Read the model definition and answer for the solid it produces. Units are mm, in the model's axes. A direction names the side the tool comes from. Coordinates: 2 decimals unless noted, no trailing zeros. Loops run counter-clockwise (first coordinate to the right, second up) from the corner with the lowest first, then second, coordinate; pieces in that order, holes last.
Q1. The mould has two halves that part along Y. Classify faces 4 (the face through (105.966, 292.984, 121.478)), 5 (the face through (205.07, -8.67, -39.05)), 6 (the face through (210, -5, 73)): pulls with the +Y half, pulls with the -Y half, needs draft (parallel to the pull), parting line crosses it, or undercut.
Q2. Section A-A (z = 0) is taken. Give the vertices of the cut face in (x, y).
Q3. Straight lines are drawn through the part: line 1 (Z direction, x = 147, y = 0); line 2 (X direction, y = 305.5, z = 112); line 3 (Y direction, x = 119, z = -268). For each, find the intervals that lie inside material, in ascending order.
Q4. Section C-C (x = 78) is taken. Give the vertices of the cut face in (y, z).
Q5. Flat-ended cylindrical pins translate along their axes: P1, Ø12, axis at x = 118, z = -73.5, coming from the +Y side; P2, Ø1.5, axis at y = -227.5, z = -124.5, coming from the -X side; P3, Ø2, axis at x = 63.5, y = 254.5, coming from the +Z side; P4, Ø5, axis at y = -206.5, z = 242.5, coming from the -X side. Find the tip coordinate at first contact, or state that the pin passes through.
Q6. Which of the six approach directions +Z, -Z, +X, -X, +Y, -Y give full straight-line access (tool end or side, diameter ignored) to faces 1 (the face through (174.75, -68.92, 310.36)), 2 (the face through (200, 4, -62)), 3 (the face through (0, -258, -157))?
from build123d import *

# Parameters (mm, degrees)
SKETCH2_R          = 300
CUT_EXTRUDE1_DEPTH = 200
SKETCH3_R          = 40
CUT_EXTRUDE2_DEPTH = 200


with BuildPart() as part:
    # Sketch1 → Revolve2 (revolve)
    with BuildSketch(Plane.XY):
        Polygon((0, 0), (0, 350), (12, 329.169330118), (24, 329.169330118), (36, 317.169330118), (174, 317.169330118), (186, 329.169330118), (198, 329.169330118), (210, 350), (210, 0), align=None)
    revolve(axis=Axis((210, 0, 0), (-1, 0, 0)))

    # Sketch2 → Cut-Extrude1 (cut)
    with BuildSketch(Plane.ZY):
        with Locations(Location((0, 0, 0), (0, 0, 270))):
            Circle(SKETCH2_R)
    extrude(amount=-CUT_EXTRUDE1_DEPTH, mode=Mode.SUBTRACT)

    # Sketch3 → Cut-Extrude2 (cut)
    with BuildSketch(Plane(origin=(210, 0, 0), x_dir=(0, 0, -1), z_dir=(1, 0, 0))):
        with Locations(Location((0, 0, 0), (0, 0, 90))):
            Circle(SKETCH3_R)
    extrude(amount=-CUT_EXTRUDE2_DEPTH, mode=Mode.SUBTRACT)


solid = part.part
Numbers:
1. face 4: parting line crosses it
1. face 5: undercut
1. face 6: needs draft
2. outline: (0, -350) - (12, -329.17) - (24, -329.17) - (36, -317.17) - (174, -317.17) - (186, -329.17) - (198, -329.17) - (210, -350) - (210, -40) - (200, -40) - (200, -300) - (0, -300) - close; (0, 300) - (200, 300) - (200, 40) - (210, 40) - (210, 350) - (198, 329.17) - (186, 329.17) - (174, 317.17) - (36, 317.17) - (24, 329.17) - (12, 329.17) - (0, 350) - close
3. line 1: z = -317.17 to -300, 300 to 317.17
3. line 2: x = 0 to 27.79, 182.21 to 210
3. line 3: y = -169.62 to -134.82, 134.82 to 169.62
4. outline: circle Ø634.34 at (0, 0); hole circle Ø600 at (0, 0)
5. P1: stops at y = 309.9
5. P2: stops at x = 200
5. P3: stops at z = 190.62
5. P4: stops at x = 0
6. face 1: none
6. face 2: -X
6. face 3: +Z, -Z, -X, +Y, -Y
